Verification items for the finished model (mm, model axes). Face numbers are marked on the shaded views. A direction names the side the tool comes from. Coordinates: 2 decimals unless noted, no trailing zeros. Write each loop counter-clockwise with the first axis right and the second up, starting at its lowest first coordinate (ties: lowest second). Pieces come first, ordered by that corner, then holes. Notation, with made-up numbers: (9.5, 77) -> (42.5, 77) arc R26 ccw to (42.5, 114) -> close; hole circle Ø2 at (33, -19). An arc over 180 degrees is marked (long way). Use a Markdown table: item, result. Add a question column.
from build123d import *

# Parameters (mm, degrees)
SKETCH1_R           = 70
BOSS_EXTRUDE1_DEPTH = 20
SKETCH2_W           = 8
SKETCH2_H           = 5
CUT_EXTRUDE1_DEPTH  = 6.89
SKETCH3_R           = 13.35
BOSS_EXTRUDE2_DEPTH = 14
CHAMFER1_SIZE       = 6


with BuildPart() as part:
    # Sketch1 → Boss-Extrude1 (new body)
    with BuildSketch(Plane(origin=(0, 0, 0), x_dir=(1, 0, 0), z_dir=(0, 1, 0))):
        Circle(SKETCH1_R)
    extrude(amount=BOSS_EXTRUDE1_DEPTH)

    # Sketch2 → Cut-Extrude1 (cut)
    with BuildSketch(Plane.XZ):
        with Locations((0, 59)):
            Rectangle(SKETCH2_W, SKETCH2_H)
        Polygon((50.930435314, 24.785898385), (55.260562333, 27.285898385), (51.260562333, 34.214101615), (46.930435314, 31.714101615), align=None)
        Polygon((46.930435314, -31.714101615), (51.260562333, -34.214101615), (55.260562333, -27.285898385), (50.930435314, -24.785898385), align=None)
        Polygon((-50.930435314, -24.785898385), (-55.260562333, -27.285898385), (-51.260562333, -34.214101615), (-46.930435314, -31.714101615), align=None)
        Polygon((-46.930435314, 31.714101615), (-51.260562333, 34.214101615), (-55.260562333, 27.285898385), (-50.930435314, 24.785898385), align=None)
    extrude(amount=-CUT_EXTRUDE1_DEPTH, mode=Mode.SUBTRACT)

    # Sketch3 → Boss-Extrude2 (add)
    with BuildSketch(Plane(origin=(0, 20, 0), x_dir=(1, 0, 0), z_dir=(0, 1, 0))):
        Circle(SKETCH3_R)
    extrude(amount=BOSS_EXTRUDE2_DEPTH)

    # Chamfer1
    chamfer1_edges = [part.edges().sort_by_distance(p)[0] for p in [
        (-13.35, 20, 0),
    ]]
    chamfer(chamfer1_edges, length=CHAMFER1_SIZE)


solid = part.part
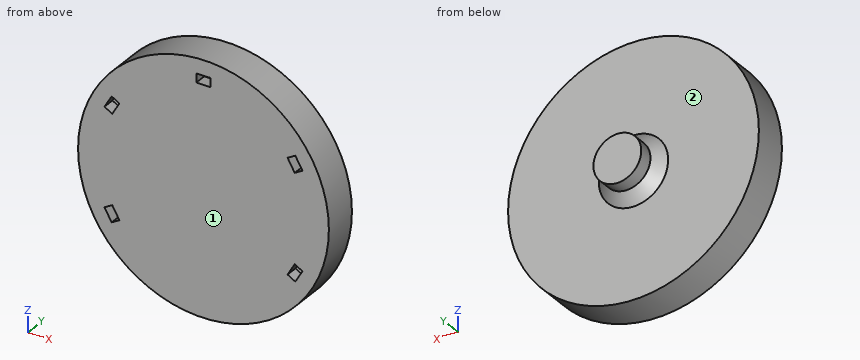
1) Cross-section at A-A on x = 0. Record the boundary of the cut face in (y, z).
2) Gauge pin test, flat ends, axial feed: pin 1 (2.5 mm diameter, centred on y = 2.5, z = 58.5, fed in from +X); pin 2 (3 mm diameter, centred on x = -10, y = 20, fed in from +Z); pin 3 (2 mm diameter, centred on x = -1, y = 3.5, fed in from -Z). Record the tip position at first contact, or that the pin passes through.
3) Cross-section at C-C on y = 28. Record the boundary of the cut face in (x, z), then the cut area to 3 significant figures.
4) Cross-section at D-D on z = -61. Record the boundary of the cut face in (x, y), then the cut area to 3 significant figures.
5) Thickness scan on L1, parallel to Y at x = -25, z = 11.5; L2, parallel to X at y = 3, z = 28; L3, parallel to X at y = 3.5, z = -25. Record the ranges inside material, lowest first.
6) Cross-section at B-B on z = 0. Record the boundary of the cut face in (x, y), then the cut area to 3 significant figures.
7) Set-up check for the marked faces 1 and 2: record each of +Z, -Z, +X, -X, +Y, -Y from which the full face is reachable in a straight line by a thin tool's end or side.
Returned:
| question | item | result |
|---|---|---|
| 1 | outline | (0, -70) -> (20, -70) -> (20, -19.35) -> (26, -13.35) -> (34, -13.35) -> (34, 13.35) -> (26, 13.35) -> (20, 19.35) -> (20, 70) -> (0, 70) -> (0, 61.5) -> (6.89, 61.5) -> (6.89, 56.5) -> (0, 56.5) -> close |
| 2 | pin 1 | stops at x = 40.28 |
| 2 | pin 2 | stops at z = 69.48 |
| 2 | pin 3 | stops at z = -70 |
| 3 | outline | circle Ø26.7 at (0, 0) |
| 3 | area | 560 mm² |
| 4 | outline | (-34.34, 0) -> (34.34, 0) -> (34.34, 20) -> (-34.34, 20) -> close |
| 4 | area | 1,370 mm² |
| 5 | L1 | y = 0 to 20 |
| 5 | L2 | x = -64.16 to -54.85, -49.07 to 49.07, 54.85 to 64.16 |
| 5 | L3 | x = -65.38 to -51.3, -50.81 to 50.81, 51.3 to 65.38 |
| 6 | outline | (-70, 0) -> (70, 0) -> (70, 20) -> (19.35, 20) -> (13.35, 26) -> (13.35, 34) -> (-13.35, 34) -> (-13.35, 26) -> (-19.35, 20) -> (-70, 20) -> close |
| 6 | area | 3,210 mm² |
| 7 | face 1 | +Z, -Z, +X, -X, -Y |
| 7 | face 2 | +Y |
